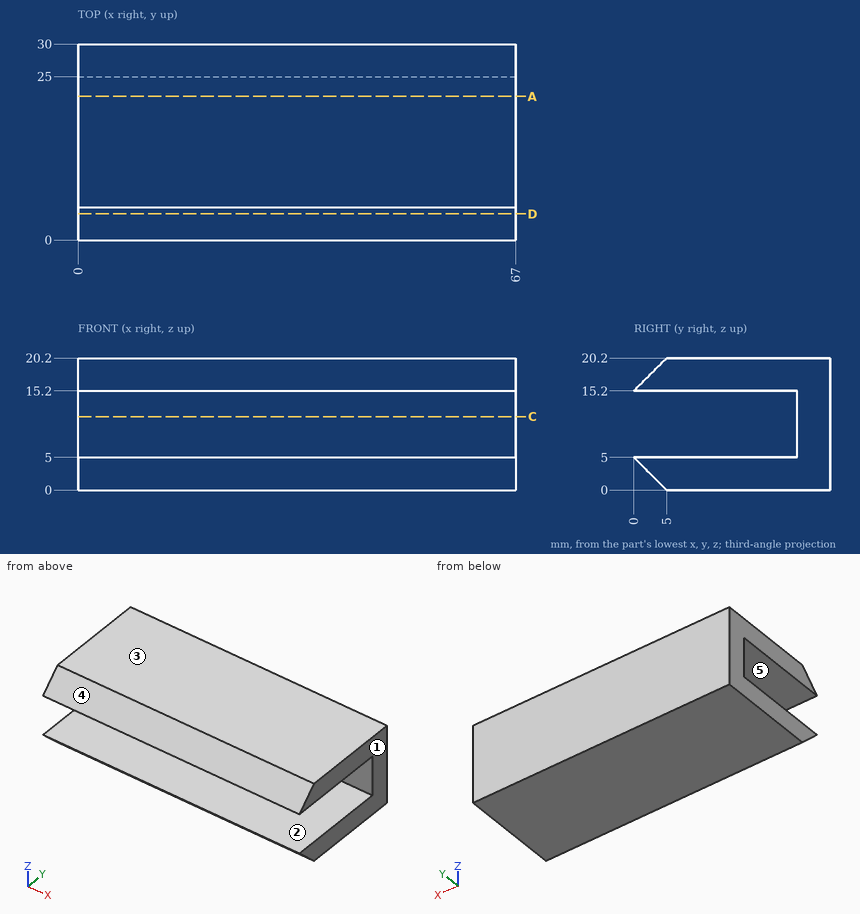
Can you work these out from the drawing? Everything is in mm from the part's minimum corner. A direction names the side the tool comes from. Round coordinates to 2 decimals unless told otherwise and drop trailing zeros. Loops run counter-clockwise (first coordinate to the right, second up) from the corner with the lowest first, then second, coordinate; pieces in that order, holes last. Notation, with made-up numbers: (50.25, 33.25) -> (54.25, 33.25) arc R23 cw to (54.25, 66.25) -> close; hole circle Ø3 at (11, 88.5). An arc over 180 degrees is marked (long way). One line per question, with ' | ' between items.
(1) If we section it at A-A on y = 22: List the corners of the cut face in (x, z) for me, and give its area (3 significant figures).
Model answer:
outline: (0, 0) -> (67, 0) -> (67, 5) -> (0, 5) -> close; (0, 15.2) -> (67, 15.2) -> (67, 20.2) -> (0, 20.2) -> close | area: 670 mm^2
(2) If we section it at D-D on y = 4: List the corners of the cut face in (x, z) for me.
Model answer:
outline: (0, 1) -> (67, 1) -> (67, 5) -> (0, 5) -> close; (0, 15.2) -> (67, 15.2) -> (67, 19.2) -> (0, 19.2) -> close
(3) For pin 1 Ø2 at (x, z) = (14, 12) entering from -Y, with a flat end and sliding along its axis, tell me the tip position at first contact or that it passes through.
Model answer:
pin 1: stops at y = 25
(4) For the marked faces 4 and 5, which set-ups out of +Z, -Z, +X, -X, +Y, -Y let a thin tool reach every point of the face, with its end or its side?
Model answer:
face 4: +Z, +X, -X, -Y | face 5: +X, -X, -Y
(5) If I drill on probe 1 along Z at (x, y) = (30.5, 18.5); probe 2 along Y at (x, z) = (5.5, 11.25); probe 3 along Y at (x, z) = (33, 4.5), over which ranges is the centre line in solid material (lowest first)?
Model answer:
probe 1: z = 0 to 5, 15.2 to 20.2 | probe 2: y = 25 to 30 | probe 3: y = 0.5 to 30
(6) If we section it at C-C on z = 11.25: List the corners of the cut face in (x, y) for me, and give its area (3 significant figures).
Model answer:
outline: (0, 25) -> (67, 25) -> (67, 30) -> (0, 30) -> close | area: 335 mm^2
(7) Thinking about a two-plate mould opening in Z: for the marked faces 1, 2 and 3, which applies, released by +Z, released by -Z, zero draft, split by the parting line, or undercut?
Model answer:
face 1: zero draft | face 2: undercut | face 3: released by +Z
